Answer from the drawing. Dimensions are ordinates in mm from the lowest x, y and z of the part. Coordinates: 2 decimals unless noted, no trailing zeros. Write each loop counter-clockwise with the first axis right and the second up, starting at its lowest first coordinate (ties: lowest second). Pieces come first, ordered by that corner, then holes. Notation, with made-up numbers: (-19, 7.5) -> (17, 7.5) arc R14 cw to (17, 22.5) -> close; hole circle Ø11 at (15, 56). An arc over 180 degrees is marked (long way). Return JSON: item names as keys, results as strings.
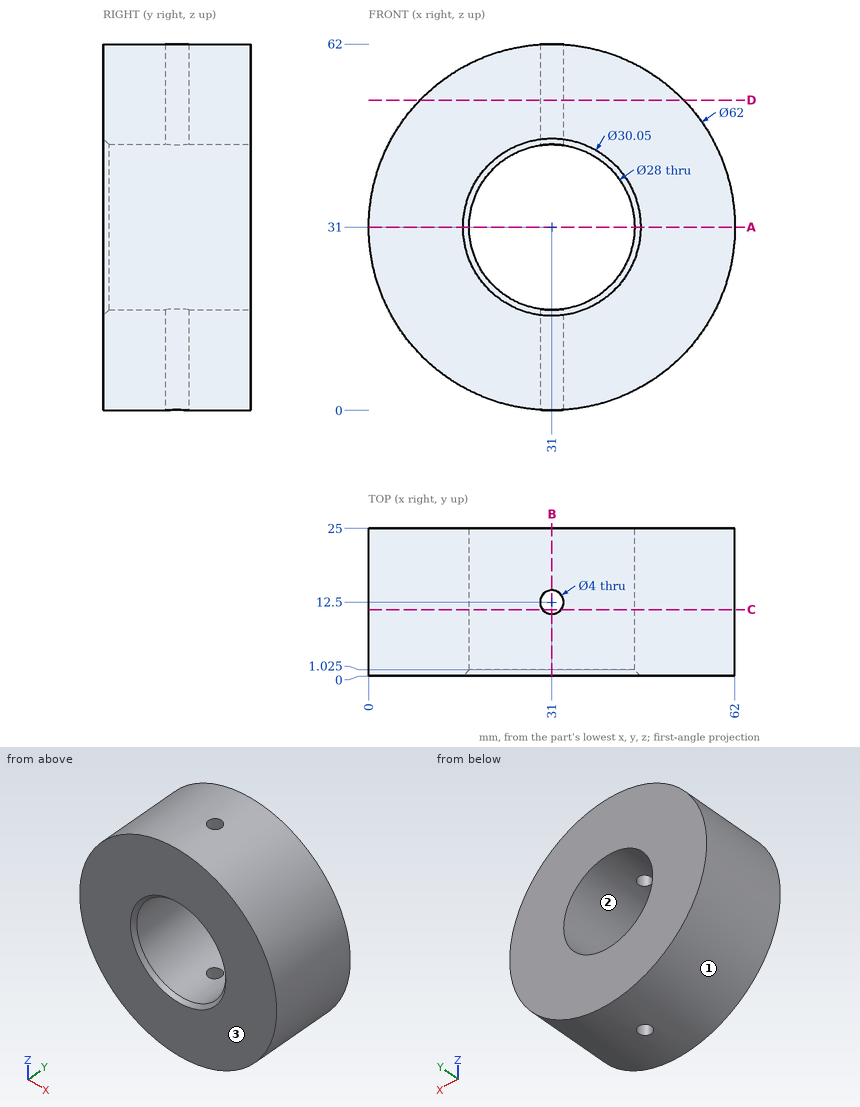
1. Flat-ended cylindrical pins translate along their axes: pin 1 Ø6 at (y, z) = (16, 43) entering from +X; pin 2 Ø1 at (x, y) = (19.5, 14) entering from +Z; pin 3 Ø6 at (y, z) = (7.5, 35.5) entering from -X. Find the tip coordinate at first contact, or state that the pin passes through.
Taken from the geometry:
{"pin 1": "stops at x = 60.66", "pin 2": "stops at z = 59.98", "pin 3": "stops at x = 0.04"}
2. The part is cut by section D-D (z = 52.5). Determine the outline of the cut face in (x, y), then the cut area to 3 significant figures.
Taken from the geometry:
{"outline": "(8.67, 0) -> (53.33, 0) -> (53.33, 25) -> (8.67, 25) -> close; hole circle Ø4 at (31, 12.5)", "area": "1,100 mm2"}
3. The part is cut by section C-C (y = 11.25). Determine the outline of the cut face in (x, z).
Taken from the geometry:
{"outline": "(29.44, 0.04) -> (29.44, 17.09) arc R14 cw to (29.44, 44.91) -> (29.44, 61.96) arc R31 ccw to start; (32.56, 0.04) arc R31 ccw to (32.56, 61.96) -> (32.56, 44.91) arc R14 cw to (32.56, 17.09) -> close"}
4. For a pull along X with two mould halves and no side action, classify the marked faces 1, 2 and 3 as +X half, -X half, draft (parallel to the pull), parting line (faces both ways), or undercut.
Taken from the geometry:
{"face 1": "parting line", "face 2": "undercut", "face 3": "draft"}
5. The part is cut by section B-B (x = 31). Determine the outline of the cut face in (y, z) (3 decimals).
Taken from the geometry:
{"outline": "(0, 0) -> (10.5, 0) -> (10.5, 17) -> (1.025, 17) -> (0, 15.975) -> close; (0, 46.025) -> (1.025, 45) -> (10.5, 45) -> (10.5, 62) -> (0, 62) -> close; (14.5, 0) -> (25, 0) -> (25, 17) -> (14.5, 17) -> close; (14.5, 45) -> (25, 45) -> (25, 62) -> (14.5, 62) -> close"}
6. The part is cut by section A-A (z = 31). Determine the outline of the cut face in (x, y) (3 decimals).
Taken from the geometry:
{"outline": "(0, 0) -> (15.975, 0) -> (17, 1.025) -> (17, 25) -> (0, 25) -> close; (45, 1.025) -> (46.025, 0) -> (62, 0) -> (62, 25) -> (45, 25) -> close"}
7. Consider L1, parallel to Y at x = 31, z = 50; L2, parallel to X at y = 8.25, z = 31.5; L3, parallel to Z at x = 21.5, y = 16. Determine where each line is inside the solid, lowest interval first.
Taken from the geometry:
{"L1": "y = 0 to 10.5, 14.5 to 25", "L2": "x = 0 to 17.01, 44.99 to 62", "L3": "z = 1.49 to 20.72, 41.28 to 60.51"}
